Input: dimensioned drawing with shaded views. Units: mm. Origin: part minimum x, y, z. Round coordinates to 2 decimals unless told otherwise and drop trailing zeros. Loops run counter-clockwise (first coordinate to the right, second up) from the corner with the lowest first, then second, coordinate; pieces in that order, holes last. Notation, with made-up numbers: M 17,-10 L 47,-10 A17 cw 47,9 Z; hole C 70.5,-16.5 d3. An arc over 180 degrees is marked long. Answer as a JSON object with one key per item and string values.
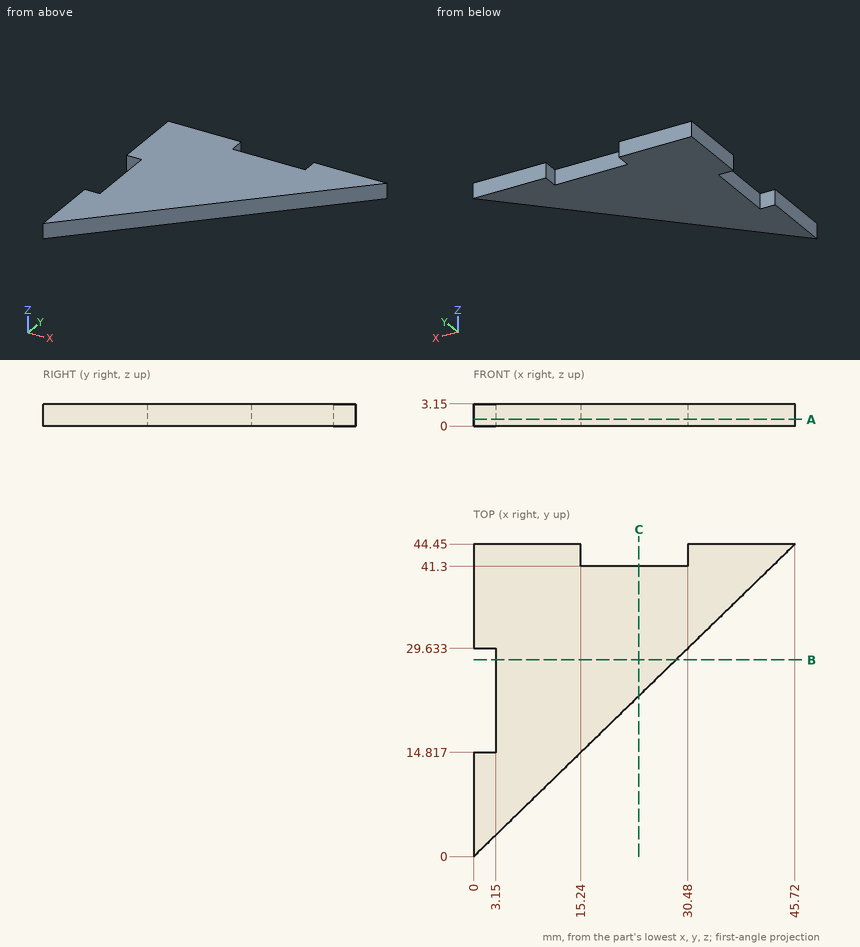
Item 1: Line query: probe 1 along X at (y, z) = (4, 1.3) (1 decimal); probe 2 along X at (y, z) = (27, 1.05); probe 3 along Y at (x, z) = (33.5, 3). Output: solid intervals per line, ascending. Write a range as from..to.
Answer sheet:
{"probe 1": "x = 0..4.1", "probe 2": "x = 3.15..27.77", "probe 3": "y = 32.57..44.45"}
Item 2: Section B-B on y = 28. Return the cut outline in (x, z).
Answer sheet:
{"outline": "M 3.15,0 L 28.8,0 L 28.8,3.15 L 3.15,3.15 Z"}
Item 3: Section C-C on x = 23.5. Return the cut outline in (y, z).
Answer sheet:
{"outline": "M 22.85,0 L 41.3,0 L 41.3,3.15 L 22.85,3.15 Z"}
Item 4: Section A-A on z = 0.95. Return the cut outline in (x, y).
Answer sheet:
{"outline": "M 0,0 L 45.72,44.45 L 30.48,44.45 L 30.48,41.3 L 15.24,41.3 L 15.24,44.45 L 0,44.45 L 0,29.63 L 3.15,29.63 L 3.15,14.82 L 0,14.82 Z"}
Item 5: Contact query for flat-ended pins moving along their axis: pin 1 Ø1.6 at (x, z) = (1.5, 1.5) entering from -Y; pin 2 Ø0.9 at (y, z) = (20, 1.5) entering from -X; pin 3 Ø10 at (x, y) = (10, 36) entering from -Z. Output: stop coordinate, or through.
Answer sheet:
{"pin 1": "stops at y = 0.68", "pin 2": "stops at x = 3.15", "pin 3": "stops at z = 0"}
